from build123d import *

# Parameters (mm, degrees)
ESQUISSE2_W = 1.25
ESQUISSE2_H = 16


with BuildPart() as part:
    # Esquisse1 → Révolution1 (revolve)
    with BuildSketch(Plane.XY, mode=Mode.PRIVATE) as r_volution1_sk:
        with BuildLine():
            Line((-5.6, 2), (-5.6, 5.5))
            Line((-5.6, 5.5), (-1.6, 5.5))
            Line((-1.6, 5.5), (-1.6, 16))
            ThreePointArc((-1.6, 16), (0, 14.4), (1.6, 16))
            Line((1.6, 16), (1.6, 2))
            Line((1.6, 2), (-5.6, 2))
        make_face()
    revolve(r_volution1_sk.sketch.rotate(Axis((-24.04155074, 0, 0), (1, 0, 0)), 90), axis=Axis((-24.04155074, 0, 0), (1, 0, 0)))

    # Esquisse2 → Trou taraudé M3x0.51 (revolve, cut)
    with BuildSketch(Plane.YZ.offset(-3.6)):
        with Locations((0.625, 8)):
            Rectangle(ESQUISSE2_W, ESQUISSE2_H)
    revolve(axis=Axis((-3.6, 0, -6.35), (0, 0, 1)), mode=Mode.SUBTRACT)


solid = part.part
Geometry check sheet. Reference: the model listing, model coordinates, mm. A direction names the side the tool comes from. Round coordinates to 2 decimals unless told otherwise and drop trailing zeros. Loops run counter-clockwise (first coordinate to the right, second up) from the corner with the lowest first, then second, coordinate; pieces in that order, holes last. Notation, with made-up numbers: (65, 57) - (122, 57) arc R34 ccw to (122, 96) - close; hole circle Ø10 at (30.25, -22). An arc over 180 degrees is marked (long way). Answer as CSV lines item,"result".
(1) Cross-section at A-A, the plane z = 0. Enter the section's corners in (x, y).
Output values:
outline,"(-5.6, -5.5) - (-1.6, -5.5) - (-1.6, -16) arc R1.6 cw to (1.6, -16) - (1.6, -2) - (-5.6, -2) - close; (-5.6, 2) - (1.6, 2) - (1.6, 16) arc R1.6 cw to (-1.6, 16) - (-1.6, 5.5) - (-5.6, 5.5) - close"
(2) Release check for a two-part mould opening along Z. For faces 1 (the face through (-2, 0, -2)), 2 (the face through (-3.57, 5.37, -1.19)), 3 (the face through (-3.65, -1.25, 3.56)) record: released by +Z, released by -Z, zero draft, split by the parting line, or undercut.
Output values:
face 1,"undercut"
face 2,"split by the parting line"
face 3,"zero draft"
(3) Cross-section at B-B, the plane y = 0. Enter the section's corners in (x, z), and give its area (3 significant figures).
Output values:
outline,"(-5.6, -5.5) - (-1.6, -5.5) - (-1.6, -16) arc R1.6 cw to (1.6, -16) - (1.6, -2) - (-5.6, -2) - close; (-5.6, 2) - (-4.85, 2) - (-4.85, 5.5) - (-5.6, 5.5) - close; (-2.35, 2) - (1.6, 2) - (1.6, 16) arc R1.6 cw to (-1.6, 16) - (-1.6, 5.5) - (-2.35, 5.5) - close"
area,"101 mm²"
(4) Depth check by flat-ended pin: pin 1 Ø2 at (x, y) = (-3.5, -8) entering from -Z; pin 2 Ø3 at (x, y) = (-5, 5.5) entering from -Z. Enter the tip coordinate at first touch or a pass-through.
Output values:
pin 1,"passes through"
pin 2,"stops at z = -3.77"
(5) Material ranges on line 1 along Y through (x, z) = (-1.75, 0); line 2 along X through (y, z) = (-9, 5); line 3 along Y through (x, z) = (-3.6, 4.6), recorded low to high.
Output values:
line 1,"y = -5.5 to -2, 2 to 5.5"
line 2,"x = -1.6 to 1.6"
line 3,"y = -3.01 to -1.25, 1.25 to 3.01"
(6) Cross-section at D-D, the plane x = -3.6. Enter the section's corners in (y, z).
Output values:
outline,"(-1.25, 1.56) - (-1.25, 5.36) arc R5.5 ccw (long way) to (1.25, 5.36) - (1.25, 1.56) arc R2 cw (long way) to start"
(7) Cross-section at C-C, the plane x = 0. Enter the section's corners in (y, z).
Output values:
outline,"circle Ø28.8 at (0, 0); hole circle Ø4 at (0, 0)"
(8) Set-up check for faces 4 (the face through (1.6, 3, 0)), 5 (the face through (-1.6, 0, -7)): record each of +Z, -Z, +X, -X, +Y, -Y from which the full face is reachable in a straight line by a thin tool's end or side.
Output values:
face 4,"+Z, -Z, +X, +Y, -Y"
face 5,"-X"
